Autodesk Inventor part; units mm, degrees
ref_plane "YZ Plane" through (0, 0, 0) normal (1, 0, 0) x (0, 1, 0)
ref_plane "XZ Plane" through (0, 0, 0) normal (0, 1, 0) x (-1, 0, 0)
ref_plane "XY Plane" through (0, 0, 0) normal (0, 0, 1) x (1, 0, 0)
sketch "Sketch1" plane through (0, 0, 0) normal (0, 1, 0) x (-1, 0, 0)
  line L0 (0, 0) -> (0, -95)
  line L1 (0, -95) -> (-95, -95)
  line L2 (-95, -95) -> (-95, -70)
  line L3 (-95, -70) -> (-25, -70)
  line L4 (-25, -70) -> (-25, 0)
  line L5 (-25, 0) -> (0, 0)
  circle A0 centre (-12.5, -20) radius 2.75
  line L6 (-12.5, 0) -> (-12.5, -95) construction
  circle A1 centre (-12.5, -40) radius 2.75
  circle A2 centre (-12.5, -60) radius 2.75
  line L7 (-95, -82.5) -> (0, -82.5) construction
  circle A3 centre (-35, -82.5) radius 2.75
  circle A4 centre (-55, -82.5) radius 2.75
  circle A5 centre (-75, -82.5) radius 2.75
  circle A6 centre (-12.5, -30) radius 2.75
  circle A7 centre (-12.5, -50) radius 2.75
  circle A8 centre (-12.5, -70) radius 2.75
  dimension "d0" = 25
  dimension "d1" = 70
  dimension "d2" = 25
  dimension "d3" = 70
  dimension "d4" = 5.5
  dimension "d5" = 20
  dimension "d6" = 5.5
  dimension "d7" = 5.5
  dimension "d8" = 20
  dimension "d9" = 20
  dimension "d12" = 5.5
  dimension "d13" = 35
  dimension "d14" = 5.5
  dimension "d15" = 20
  dimension "d16" = 5.5
  dimension "d17" = 20
  dimension "d22" = 10
extrude "Extrusion1" add sketch "Sketch1" along normal blind 4
fillet "Fillet1" radius 20 1 edges at (25, 2, -70)
properties part number "Brace 1" material "CFRP"
Check sheet for the modelled part. Datum: model origin and axes. Units: mm. A direction names the side the tool comes from. Round coordinates to 2 decimals unless told otherwise and drop trailing zeros. Order: outer loops, then holes, each group sorted by start corner. A loop starts at its lowest first (then second) coordinate and runs counter-clockwise, first axis right, second up. Notation, with made-up numbers: M 49.25,59 L 71.25,59 A37 ccw 71.25,96 Z; hole C 35,22 d1. An arc over 180 degrees is marked long. Answer in a Markdown table with one row per item.
(1) Section check C-C on y = 1.7. Give the number of separate pieces and of enclosed holes in the cut face, plus the area to 3 significant figures.
Findings:
| item | result |
|---|---|
| separate pieces | 1 |
| enclosed holes | 9 |
| area | 4,000 mm^2 |
(2) Material ranges on line 1 along Z through (x, y) = (75, 1.15); line 2 along Z through (x, y) = (83, 3.05); line 3 along X through (y, z) = (0.7, -9), recorded low to high. Write a range as from..to.
Findings:
| item | result |
|---|---|
| line 1 | z = -95..-85.25, -79.75..-70 |
| line 2 | z = -95..-70 |
| line 3 | x = 0..25 |
(3) Section check B-B on z = -30. Record the boundary of the cut face in (x, y).
Findings:
| item | result |
|---|---|
| outline | M 0,0 L 9.75,0 L 9.75,4 L 0,4 Z; M 15.25,0 L 25,0 L 25,4 L 15.25,4 Z |
(4) Draft check along X on faces 3 (the cylindrical face through (31.014, 2.028, -64.297)), 4 (the cylindrical face through (12.858, 1.972, -42.727)), 5 (the flat face through (47, 2, -95)). Enter one of: +X half, -X half, draft (parallel to the pull), parting line (faces both ways), or undercut.
Findings:
| item | result |
|---|---|
| face 3 | +X half |
| face 4 | undercut |
| face 5 | draft |
(5) Section check A-A on x = 55. Record the boundary of the cut face in (y, z).
Findings:
| item | result |
|---|---|
| outline | M 0,-95 L 4,-95 L 4,-85.25 L 0,-85.25 Z; M 0,-79.75 L 4,-79.75 L 4,-70 L 0,-70 Z |
(6) Gauge pin test, flat ends, axial feed: pin 1 (2 mm diameter, centred on x = 69.5, y = 3, fed in from +Z); pin 2 (2 mm diameter, centred on y = 2, z = -19, fed in from +X). Record the tip position at first contact, or that the pin passes through.
Findings:
| item | result |
|---|---|
| pin 1 | stops at z = -70 |
| pin 2 | stops at x = 25 |
(7) Section check D-D on z = -82.5. Record the boundary of the cut face in (x, y), plus the area to 3 significant figures.
Findings:
| item | result |
|---|---|
| outline | M 0,0 L 32.25,0 L 32.25,4 L 0,4 Z; M 37.75,0 L 52.25,0 L 52.25,4 L 37.75,4 Z; M 57.75,0 L 72.25,0 L 72.25,4 L 57.75,4 Z; M 77.75,0 L 95,0 L 95,4 L 77.75,4 Z |
| area | 314 mm^2 |
(8) Set-up check for faces 1 (the cylindrical face through (12.858, 1.972, -52.727)), 2 (the flat face through (70, 2, -70)): record each of +Z, -Z, +X, -X, +Y, -Y from which the full face is reachable in a straight line by a thin tool's end or side.
Findings:
| item | result |
|---|---|
| face 1 | +Y, -Y |
| face 2 | +Z, +X, +Y, -Y |
